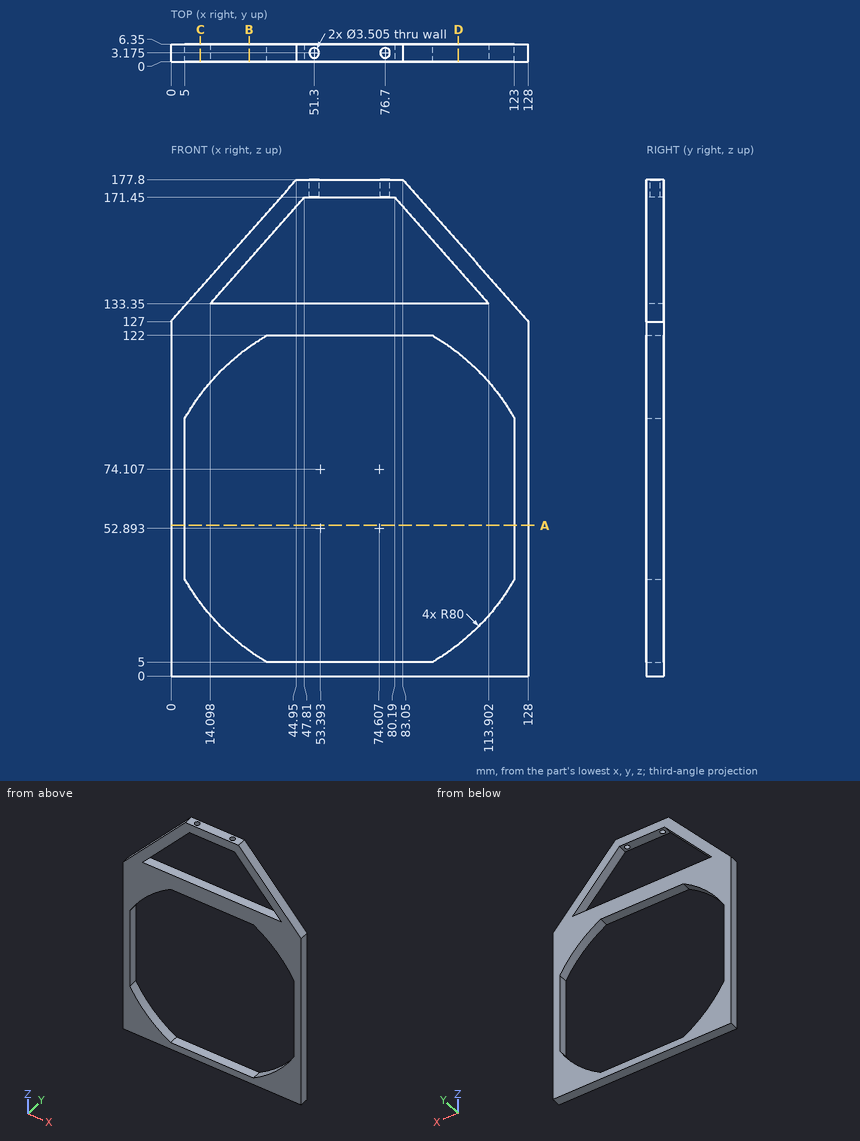
Can you work these out from the drawing? Everything is in mm from the part's minimum corner. Give positions to 0.01 mm unless a question says otherwise; leave off trailing zeros. Write each loop counter-clockwise with the first axis right and the second up, starting at its lowest first coordinate (ties: lowest second). Pieces come first, ordered by that corner, then holes. Notation, with made-up numbers: (85, 68.5) -> (133, 68.5) arc R21 cw to (133, 83.5) -> close; hole circle Ø2 at (-23.5, 84). An arc over 180 degrees is marked (long way). Write each question's results on one line, items separated by ' | '. Start each with the question number.
Q1. I need wall thicknesses on probe 1 along Z at (x, y) = (70.5, 5.75); probe 2 along Y at (x, z) = (51, 174); probe 3 along X at (y, z) = (5.5, 73.5). Which ranges of each line are inside material? Lowest first, please.
Q2. Suppose I cut it at D-D, the plane x = 103. List the corners of the cut face in (y, z) for me.
Q3. I'm going to push flat-ended pins straight in: pin 1 Ø1.5 at (y, z) = (3.5, 134.5) entering from +X; pin 2 Ø1 at (y, z) = (4.5, 157) entering from -X; pin 3 Ø3 at (y, z) = (5, 148) entering from -X (1 decimal). Where does each tip first touch, or does it pass through?
Q4. Suppose I cut it at B-B, the plane x = 28. State how many separate pieces and enclosed holes the cut face has.
Q5. Suppose I cut it at C-C, the plane x = 10.5. List the corners of the cut face in (y, z) for me, and give its area (3 significant figures).
Q6. Suppose I cut it at A-A, the plane z = 54. List the corners of the cut face in (x, y) for me, and give its area (3 significant figures).
Outcome:
1) probe 1: 0 to 5, 122 to 133.35, 171.45 to 177.8 | probe 2: 0 to 1.45, 4.9 to 6.35 | probe 3: 0 to 5, 123 to 128
2) outline: (0, 0) -> (6.35, 0) -> (6.35, 11.34) -> (0, 11.34) -> close; (0, 115.66) -> (6.35, 115.66) -> (6.35, 133.35) -> (0, 133.35) -> close; (0, 145.67) -> (6.35, 145.67) -> (6.35, 155.25) -> (0, 155.25) -> close
3) pin 1: x = 122.03 | pin 2: x = 26.1 | pin 3: x = 17.3
4) separate pieces: 3 | enclosed holes: 0
5) outline: (0, 0) -> (6.35, 0) -> (6.35, 26.25) -> (0, 26.25) -> close; (0, 100.75) -> (6.35, 100.75) -> (6.35, 138.87) -> (0, 138.87) -> close | area: 409 mm2
6) outline: (0, 0) -> (5, 0) -> (5, 6.35) -> (0, 6.35) -> close; (123, 0) -> (128, 0) -> (128, 6.35) -> (123, 6.35) -> close | area: 63.5 mm2
